Input: part model. Units: mm. Frame: model coordinates. Face numbers are marked on the shaded views. A direction names the side the tool comes from. Give positions to 0.01 mm unless a question says otherwise; leave off trailing zeros. Write each loop counter-clockwise with the first axis right and the second up, starting at its lowest first coordinate (ties: lowest second). Pieces come first, ordered by that corner, then holes. Notation, with made-up numbers: (22.25, 28) -> (65.25, 28) arc R24 ccw to (65.25, 66) -> close; hole circle Ø4 at (58.25, 64.25). An arc over 180 degrees is marked (long way). Answer as a JSON object with one key per item and string values. Group by question number.
from build123d import *
from build123d import SkipClean  # not in build123d's __all__

# Parameters (mm, degrees)
F0_R     = 0.75
F0_R_2   = 0.5
F1_DEPTH = 2.1
F2_R     = 1.85
F3_DEPTH = 1.5
F4_R     = 2.55
F4_R_2   = 2.05
F5_DEPTH = 1


# Not quite as in the source:
# - after a boolean that leaves OpenCascade's solid faulty, fix() repairs it


with BuildPart() as f1:
    # F0 (on Top) → F1 (new body)
    with BuildSketch(Plane.XY):
        with BuildLine():
            ThreePointArc((-2.9169642705, 0.2166666667), (-0.108407815, -2.9229903773), (2.925, 0))
            ThreePointArc((2.925, 0), (2.9229903773, 0.108407815), (2.9169642705, 0.2166666667))
            ThreePointArc((2.9169642705, 0.2166666667), (0, 2.925), (-2.9169642705, 0.2166666667))
        make_face()
        Circle(F0_R, mode=Mode.SUBTRACT)
        with BuildLine():
            ThreePointArc((-2.9169642705, 0.2166666667), (0, 2.925), (2.9169642705, 0.2166666667))
            Line((2.9169642705, 0.2166666667), (1.9197115285, 13.6425925926))
            ThreePointArc((1.9197115285, 13.6425925926), (1.9236774278, 13.5713453141), (1.925, 13.5))
            ThreePointArc((1.925, 13.5), (-0.0713453141, 11.5763225722), (-1.9197115285, 13.6425925926))
            Line((-1.9197115285, 13.6425925926), (-2.9169642705, 0.2166666667))
        make_face()
        with BuildLine():
            ThreePointArc((1.925, 13.5), (1.9236774278, 13.5713453141), (1.9197115285, 13.6425925926))
            ThreePointArc((1.9197115285, 13.6425925926), (0, 15.425), (-1.9197115285, 13.6425925926))
            ThreePointArc((-1.9197115285, 13.6425925926), (-0.0713453141, 11.5763225722), (1.925, 13.5))
        make_face()
        with Locations((0, 13.5)):
            Circle(F0_R_2, mode=Mode.SUBTRACT)
    extrude(amount=F1_DEPTH)

    # F2 (on face) → F3 (join)
    with BuildSketch(Plane.XY):
        with BuildLine():
            ThreePointArc((2.9169642705, 0.2166666667), (0, 2.925), (-2.9169642705, 0.2166666667))
            ThreePointArc((-2.9169642705, 0.2166666667), (0, -2.925), (2.9169642705, 0.2166666667))
        make_face()
        Circle(F2_R, mode=Mode.SUBTRACT)
    with SkipClean():  # cleaning this boolean's faces spoils the solid; the shape is the same uncleaned
        extrude(amount=-F3_DEPTH)

    # F4 (on face) → F5 (join)
    with BuildSketch(Plane.XY.offset(2.1)):
        Circle(F4_R)
        Circle(F4_R_2, mode=Mode.SUBTRACT)
    extrude(amount=F5_DEPTH)

    add(f1.part.fix(), mode=Mode.REPLACE)


solid = f1.part
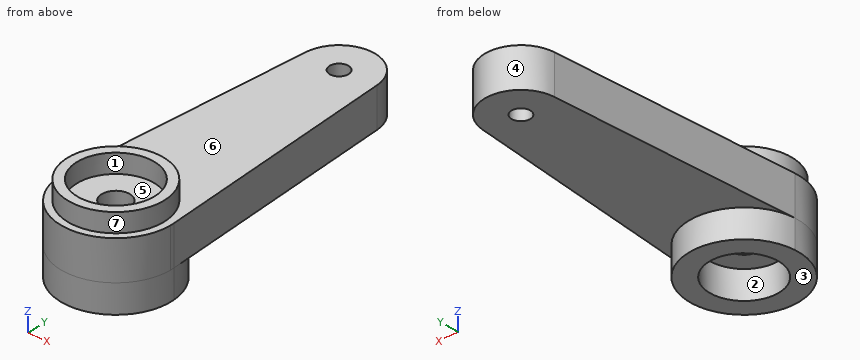
1. Section D-D (z = -0.2). Return the cut outline in (x, y) (3 decimals).
2. Section A-A (z = 0.5). Return the cut outline in (x, y) (3 decimals), plus the area to 3 significant figures.
3. Section C-C (x = 2.25). Return the cut outline in (y, z), plus the area to 3 significant figures.
4. Contact query for flat-ended pins moving along their axis: pin 1 Ø1.5 at (y, z) = (1.5, -0.5) entering from -X; pin 2 Ø3.5 at (x, y) = (0, 0) entering from +Z; pin 3 Ø1.7 at (x, y) = (0, 0) entering from -Z. Output: stop coordinate, or through.
5. Mould query, pull axis Y, two halves, no side actions, for the marked faces 4, 5, 6 and 7. Classes: pulls with the +Y half, pulls with the -Y half, needs draft (parallel to the pull), parting line crosses it, or undercut.
6. Section B-B (x = 0). Return the cut outline in (y, z) (3 decimals).
7. Line query: line 1 (Y direction, x = 0, z = 0.45) (3 decimals); line 2 (Z direction, x = 1.95, y = -0.5); line 3 (Z direction, x = 1.25, y = 6.5). Output: solid intervals per line, ascending.
8. Reachability of the marked faces 1, 2 and 3 from +Z, -Z, +X, -X, +Y, -Y: full face, straight path, thin tool, end or side. Return the list, or none.
Working result:
{
 "1": {"outline": "circle Ø5.85 at (0, 0); hole circle Ø3.7 at (0, 0)"},
 "2": {"outline": "(-2.917, 0.217) arc R2.925 ccw (long way) to (2.917, 0.217) -> (1.92, 13.643) arc R1.925 ccw to (-1.92, 13.643) -> close; hole circle Ø1.5 at (0, 0); hole circle Ø1 at (0, 13.5)", "area": "82.4 mm^2"},
 "3": {"outline": "(-1.87, -1.5) -> (1.87, -1.5) -> (1.87, 0) -> (9.2, 0) -> (9.2, 2.1) -> (1.2, 2.1) -> (1.2, 3.1) -> (-1.2, 3.1) -> (-1.2, 2.1) -> (-1.87, 2.1) -> close", "area": "31.2 mm^2"},
 "4": {"pin 1": "stops at x = -2.86", "pin 2": "stops at z = 2.1", "pin 3": "stops at z = 0"},
 "5": {"face 4": "pulls with the +Y half", "face 5": "undercut", "face 6": "needs draft", "face 7": "parting line crosses it"},
 "6": {"outline": "(-2.925, -1.5) -> (-1.85, -1.5) -> (-1.85, 0) -> (-0.75, 0) -> (-0.75, 2.1) -> (-2.05, 2.1) -> (-2.05, 3.1) -> (-2.55, 3.1) -> (-2.55, 2.1) -> (-2.925, 2.1) -> close; (0.75, 0) -> (1.85, 0) -> (1.85, -1.5) -> (2.925, -1.5) -> (2.925, 0) -> (13, 0) -> (13, 2.1) -> (2.55, 2.1) -> (2.55, 3.1) -> (2.05, 3.1) -> (2.05, 2.1) -> (0.75, 2.1) -> close; (14, 0) -> (15.425, 0) -> (15.425, 2.1) -> (14, 2.1) -> close"},
 "7": {"line 1": "y = -2.925 to -0.75, 0.75 to 13, 14 to 15.425", "line 2": "z = -1.5 to 2.1", "line 3": "z = 0 to 2.1"},
 "8": {"face 1": "+Z", "face 2": "-Z", "face 3": "-Z, +X, -X, +Y, -Y"}
}
